```python
from build123d import *

# Parameters (mm, degrees)
CROQUIS1_W              = 100
CROQUIS1_H              = 150
SALIENTE_EXTRUIR1_DEPTH = 2
CROQUIS5_W              = 100
CROQUIS5_H              = 150
CROQUIS5_W_2            = 94
CROQUIS5_H_2            = 144
SALIENTE_EXTRUIR3_DEPTH = 15
CROQUIS6_W              = 20
CROQUIS6_H              = 20
SALIENTE_EXTRUIR4_DEPTH = 17
CROQUIS4_R              = 2
CORTAR_EXTRUIR2_DEPTH   = 92.378334412
SALIENTE_EXTRUIR5_DEPTH = 7.5
CROQUIS8_W              = 127.938872722
CROQUIS8_H              = 211.588515632
CROQUIS8_W_2            = 100
CROQUIS8_H_2            = 150
CORTAR_EXTRUIR3_DEPTH   = 115.867495711
CORTAR_EXTRUIR4_DEPTH   = 7.5
CROQUIS10_W             = 60
CROQUIS10_H             = 1.5
CROQUIS10_W_2           = 1.5
CROQUIS10_H_2           = 110
SALIENTE_EXTRUIR6_DEPTH = 3
CROQUIS12_R             = 0.6
CORTAR_EXTRUIR5_DEPTH   = 2
CORTAR_EXTRUIR7_DEPTH   = 157.655827733


with BuildPart() as part:
    # Croquis1 → Saliente-Extruir1 (new body)
    with BuildSketch(Plane(origin=(0, 0, 0), x_dir=(1, 0, 0), z_dir=(0, 1, 0))):
        Rectangle(CROQUIS1_W, CROQUIS1_H)
    extrude(amount=SALIENTE_EXTRUIR1_DEPTH)

    # Croquis5 → Saliente-Extruir3 (add)
    with BuildSketch(Plane(origin=(0, 2, 0), x_dir=(1, 0, 0), z_dir=(0, 1, 0))):
        Rectangle(CROQUIS5_W, CROQUIS5_H)
        Rectangle(CROQUIS5_W_2, CROQUIS5_H_2, mode=Mode.SUBTRACT)
    extrude(amount=SALIENTE_EXTRUIR3_DEPTH)

    # Croquis6 → Saliente-Extruir4 (add)
    with BuildSketch(Plane.XZ):
        with Locations((-40, 65)):
            Rectangle(CROQUIS6_W, CROQUIS6_H)
        with Locations((-40, -65)):
            Rectangle(CROQUIS6_W, CROQUIS6_H)
        with Locations((40, -65)):
            Rectangle(CROQUIS6_W, CROQUIS6_H)
        with Locations((40, 65)):
            Rectangle(CROQUIS6_W, CROQUIS6_H)
    extrude(amount=-SALIENTE_EXTRUIR4_DEPTH)

    # Croquis4 → Cortar-Extruir2 (cut, through all)
    # profile 1 of 4: a face of its own
    with BuildSketch(Plane(origin=(0, 2, 0), x_dir=(1, 0, 0), z_dir=(0, 1, 0))):
        with BuildLine():
            Line((-44.924038765, 64.131759112), (-46.660520542, 73.979836642))
            ThreePointArc((-46.660520542, 73.979836642), (-42.604722665, 79.772116295), (-36.812443012, 75.716318418))
            Line((-36.812443012, 75.716318418), (-35.075961235, 65.868240888))
            ThreePointArc((-35.075961235, 65.868240888), (-39.131759112, 60.075961235), (-44.924038765, 64.131759112))
        make_face()
        with Locations(Location((-40, 65, 0), (0, 0, 90))):
            Circle(CROQUIS4_R, mode=Mode.SUBTRACT)
    # profile 2 of 4: a face of its own
    with BuildSketch(Plane(origin=(0, 2, 0), x_dir=(1, 0, 0), z_dir=(0, 1, 0))):
        with BuildLine():
            Line((44.924038765, -64.131759112), (46.660520542, -73.979836642))
            ThreePointArc((46.660520542, -73.979836642), (42.604722665, -79.772116295), (36.812443012, -75.716318418))
            Line((36.812443012, -75.716318418), (35.075961235, -65.868240888))
            ThreePointArc((35.075961235, -65.868240888), (39.131759112, -60.075961235), (44.924038765, -64.131759112))
        make_face()
        with Locations(Location((40, -65, 0), (0, 0, 90))):
            Circle(CROQUIS4_R, mode=Mode.SUBTRACT)
    # profile 3 of 4: a face of its own
    with BuildSketch(Plane(origin=(0, 2, 0), x_dir=(1, 0, 0), z_dir=(0, 1, 0))):
        with BuildLine():
            Line((44.924038765, 64.131759112), (46.660520542, 73.979836642))
            ThreePointArc((46.660520542, 73.979836642), (42.604722665, 79.772116295), (36.812443012, 75.716318418))
            Line((36.812443012, 75.716318418), (35.075961235, 65.868240888))
            ThreePointArc((35.075961235, 65.868240888), (39.131759112, 60.075961235), (44.924038765, 64.131759112))
        make_face()
        with Locations(Location((40, 65, 0), (0, 0, 90))):
            Circle(CROQUIS4_R, mode=Mode.SUBTRACT)
    # profile 4 of 4: a face of its own
    with BuildSketch(Plane(origin=(0, 2, 0), x_dir=(1, 0, 0), z_dir=(0, 1, 0))):
        with BuildLine():
            Line((-44.924038765, -64.131759112), (-46.660520542, -73.979836642))
            ThreePointArc((-46.660520542, -73.979836642), (-42.604722665, -79.772116295), (-36.812443012, -75.716318418))
            Line((-36.812443012, -75.716318418), (-35.075961235, -65.868240888))
            ThreePointArc((-35.075961235, -65.868240888), (-39.131759112, -60.075961235), (-44.924038765, -64.131759112))
        make_face()
        with Locations(Location((-40, -65, 0), (0, 0, 90))):
            Circle(CROQUIS4_R, mode=Mode.SUBTRACT)
    extrude(amount=CORTAR_EXTRUIR2_DEPTH, mode=Mode.SUBTRACT)

    # Croquis7 → Saliente-Extruir5 (add)
    with BuildSketch(Plane(origin=(0, 2, 0), x_dir=(1, 0, 0), z_dir=(0, 1, 0))):
        with BuildLine():
            Line((35.075961235, 65.868240888), (39.187090394, 89.183612944))
            ThreePointArc((39.187090394, 89.183612944), (44.979370047, 93.239410821), (49.035167924, 87.447131167))
            Line((49.035167924, 87.447131167), (44.924038765, 64.131759112))
            ThreePointArc((44.924038765, 64.131759112), (39.131759112, 60.075961235), (35.075961235, 65.868240888))
        make_face()
        with BuildLine():
            Line((-44.924038765, 64.131759112), (-50.51627176, 95.846888427))
            ThreePointArc((-50.51627176, 95.846888427), (-46.460473883, 101.63916808), (-40.66819423, 97.583370203))
            Line((-40.66819423, 97.583370203), (-35.075961235, 65.868240888))
            ThreePointArc((-35.075961235, 65.868240888), (-39.131759112, 60.075961235), (-44.924038765, 64.131759112))
        make_face()
        with BuildLine():
            Line((-35.075961235, -65.868240888), (-36.812443012, -75.716318418))
            ThreePointArc((-36.812443012, -75.716318418), (-42.604722665, -79.772116295), (-46.660520542, -73.979836642))
            Line((-46.660520542, -73.979836642), (-44.924038765, -64.131759112))
            ThreePointArc((-44.924038765, -64.131759112), (-39.131759112, -60.075961235), (-35.075961235, -65.868240888))
        make_face()
        with BuildLine():
            Line((44.924038765, -64.131759112), (47.53565731, -78.942983887))
            ThreePointArc((47.53565731, -78.942983887), (43.479859434, -84.73526354), (37.68757978, -80.679465664))
            Line((37.68757978, -80.679465664), (35.075961235, -65.868240888))
            ThreePointArc((35.075961235, -65.868240888), (39.131759112, -60.075961235), (44.924038765, -64.131759112))
        make_face()
    extrude(amount=SALIENTE_EXTRUIR5_DEPTH)

    # Croquis8 → Cortar-Extruir3 (cut, through all)
    with BuildSketch(Plane.XZ):
        Rectangle(CROQUIS8_W, CROQUIS8_H)
        Rectangle(CROQUIS8_W_2, CROQUIS8_H_2, mode=Mode.SUBTRACT)
    extrude(amount=-CORTAR_EXTRUIR3_DEPTH, mode=Mode.SUBTRACT)

    # Croquis9 → Cortar-Extruir4 (cut)
    with BuildSketch(Plane(origin=(0, 17, 0), x_dir=(1, 0, 0), z_dir=(0, 1, 0))):
        with BuildLine():
            Line((-50, -74.5), (-50, -75))
            Line((-50, -75), (-44.511576947, -75))
            Line((-44.511576947, -75), (-44.511576947, -62.844617563))
            add(Edge.make_bspline(
                [(-50, -74.5), (-46.388295921, -69.021503378), (-44.511576947, -62.844617563)],
                knots=[0, 0, 0, 1, 1, 1], degree=2))
        make_face()
        with BuildLine():
            Line((50, -75), (44.511576947, -75))
            Line((44.511576947, -75), (44.511576947, -62.844617563))
            add(Edge.make_bspline(
                [(50, -74.5), (46.388295921, -69.021503378), (44.511576947, -62.844617563)],
                knots=[0, 0, 0, 1, 1, 1], degree=2))
            Line((50, -74.5), (50, -75))
        make_face()
        with BuildLine():
            Line((-50, 75), (-44.511576947, 75))
            Line((-44.511576947, 75), (-44.511576947, 62.844617563))
            add(Edge.make_bspline(
                [(-50, 74.5), (-46.388295921, 69.021503378), (-44.511576947, 62.844617563)],
                knots=[0, 0, 0, 1, 1, 1], degree=2))
            Line((-50, 74.5), (-50, 75))
        make_face()
        with BuildLine():
            Line((50, 75), (44.511576947, 75))
            Line((44.511576947, 75), (44.511576947, 62.844617563))
            add(Edge.make_bspline(
                [(50, 74.5), (46.388295921, 69.021503378), (44.511576947, 62.844617563)],
                knots=[0, 0, 0, 1, 1, 1], degree=2))
            Line((50, 74.5), (50, 75))
        make_face()
    extrude(amount=-CORTAR_EXTRUIR4_DEPTH, mode=Mode.SUBTRACT)

    # Croquis10 → Saliente-Extruir6 (add)
    with BuildSketch(Plane(origin=(0, 17, 0), x_dir=(1, 0, 0), z_dir=(0, 1, 0))):
        with Locations((0, 72.75)):
            Rectangle(CROQUIS10_W, CROQUIS10_H)
        with Locations((0, -72.75)):
            Rectangle(CROQUIS10_W, CROQUIS10_H)
        with Locations((-47.75, 0)):
            Rectangle(CROQUIS10_W_2, CROQUIS10_H_2)
        with Locations((47.75, 0)):
            Rectangle(CROQUIS10_W_2, CROQUIS10_H_2)
    extrude(amount=SALIENTE_EXTRUIR6_DEPTH)

    # Croquis12 → Cortar-Extruir5 (cut)
    with BuildSketch(Plane(origin=(0, 17, 0), x_dir=(1, 0, 0), z_dir=(0, 1, 0))):
        with Locations(Location((-40, -65, 0), (0, 0, 270))):
            Circle(CROQUIS12_R)
        with Locations(Location((-40, 65, 0), (0, 0, 90))):
            Circle(CROQUIS12_R)
        with Locations(Location((40, 65, 0), (0, 0, 270))):
            Circle(CROQUIS12_R)
        with Locations(Location((40, -65, 0), (0, 0, 90))):
            Circle(CROQUIS12_R)
    extrude(amount=-CORTAR_EXTRUIR5_DEPTH, mode=Mode.SUBTRACT)

    # Croquis17 → Revolución4 (revolve)
    with BuildSketch(Plane(origin=(-12.5, 0, -12.5), x_dir=(-0.7071067811865475, 0, 0.7071067811865476), z_dir=(-0.7071067811865476, 0, -0.7071067811865475)), mode=Mode.PRIVATE) as revoluci_n4_sk:
        Polygon((-74.388347648, 5.812970012), (-139.644463954, -21.860187069), (-143.51805142, -12.725874225), (-138.914857092, -10.773797899), (-136.962780767, -15.376992227), (-77.121254504, 10), align=None)
    revoluci_n4 = revolve(revoluci_n4_sk.sketch.rotate(Axis((40.100505063, 5.812970012, -65.100505063), (0.6509899848797962, -0.3904152650350718, -0.6509899848797963)), 90), axis=Axis((40.100505063, 5.812970012, -65.100505063), (0.6509899848797962, -0.3904152650350718, -0.6509899848797963)))

    # Simetría4: Revolución4 across plane
    add(revoluci_n4.mirror(Plane.XY))

    # Simetría5: Revolución4 across plane
    add(revoluci_n4.mirror(Plane(origin=(0, 0, 0), x_dir=(0, 0, 1), z_dir=(1, 0, 0))))

    # Simetría5 copy 1 sketch → Simetría5 copy 1 (revolve)
    with BuildSketch(Plane(origin=(12.5, 0, 12.5), x_dir=(0.7071067811865475, 0, -0.7071067811865476), z_dir=(0.7071067811865476, 0, 0.7071067811865475))):
        Polygon((-74.388347648, 5.812970012), (-139.644463954, -21.860187069), (-143.51805142, -12.725874225), (-138.914857092, -10.773797899), (-136.962780767, -15.376992227), (-77.121254504, 10), align=None)
    revolve(axis=Axis((-40.100505063, 5.812970012, 65.100505063), (-0.6509899848797962, -0.3904152650350718, 0.6509899848797963)))

    # Croquis19 → Cortar-Extruir7 (cut, through all)
    with BuildSketch(Plane(origin=(0, 9.5, 0), x_dir=(1, 0, 0), z_dir=(0, 1, 0))):
        Polygon((-43.417017803, -64.899000462), (-39.692445235, -68.264184449), (-41.99457515, -70.812172899), (-45.719147718, -67.446988912), align=None)
        Polygon((39.692445235, -68.264184449), (41.99457515, -70.812172899), (45.719147718, -67.446988912), (43.417017803, -64.899000462), align=None)
        Polygon((43.417017803, 64.899000462), (39.692445235, 68.264184449), (41.99457515, 70.812172899), (45.719147718, 67.446988912), align=None)
        Polygon((-39.692445235, 68.264184449), (-41.99457515, 70.812172899), (-45.719147718, 67.446988912), (-43.417017803, 64.899000462), align=None)
    extrude(amount=CORTAR_EXTRUIR7_DEPTH, mode=Mode.SUBTRACT)


solid = part.part
```
Work out the finished part from the listing and answer in its coordinate system (mm). A direction names the side the tool comes from. Coordinates: 2 decimals unless noted, no trailing zeros. Loops run counter-clockwise (first coordinate to the right, second up) from the corner with the lowest first, then second, coordinate; pieces in that order, holes last.
1) Section A-A (x = 23.5) is taken. Give the vertices of the cut face in (y, z).
Results:
outline: (0, -75) - (17, -75) - (17, -73.5) - (20, -73.5) - (20, -72) - (2, -72) - (2, 72) - (20, 72) - (20, 73.5) - (17, 73.5) - (17, 75) - (0, 75) - close
2) Flat-ended cylindrical pins translate along their axes: pin 1 (1.6 mm diameter, centred on x = 40, z = -65, fed in from -Y); pin 2 (4.5 mm diameter, centred on x = -42.5, y = 6.5, fed in from +Z); pin 3 (12 mm diameter, centred on y = 9, z = -63, fed in from -X). Find the tip coordinate at first contact, or state that the pin passes through.
Results:
pin 1: stops at y = 0
pin 2: stops at z = 75
pin 3: stops at x = -50
3) For a pull along Y with two mould halves and no side action, classify faces 1 (the flat face through (-85.558, -22.066, 104.125)), 2 (the flat face through (-30, 9, 63)), 3 (the flat face through (86.3, -21.99, 111.11)) as +Y half, -Y half, draft (parallel to the pull), parting line (faces both ways), or undercut.
Results:
face 1: undercut
face 2: draft
face 3: -Y half
4) For faces 4 (the cylindrical face through (39, 13.2, -60.1)), 5 (the flat face through (-86.3, -21.99, -111.11)), 6 (the flat face through (-80.076, -24.096, -108.39)), determine the directions among +Z, -Z, +X, -X, +Y, -Y from which every point of the face is accessible in a straight line to the end or side of a thin tool.
Results:
face 4: +Y
face 5: -Z, -X, -Y
face 6: none
5) Section B-B (z = 4.5) is taken. Give the vertices of the cut face in (x, y), plus the area to 3 significant figures.
Results:
outline: (-50, 0) - (50, 0) - (50, 17) - (48.5, 17) - (48.5, 20) - (47, 20) - (47, 2) - (-47, 2) - (-47, 20) - (-48.5, 20) - (-48.5, 17) - (-50, 17) - close
area: 299 mm2
6) Consider probe 1 along Z at (x, y) = (6, 11.5); probe 2 along X at (y, z) = (8, -45); probe 3 along Y at (x, z) = (43.5, -11.5). Determine where each line is inside the solid, lowest interval first.
Results:
probe 1: z = -75 to -72, 72 to 75
probe 2: x = -50 to -47, 47 to 50
probe 3: y = 0 to 2
7) Section C-C (y = -8) is taken. Give the number of separate pieces and of enclosed holes in the cut face, plus the area to 3 significant figures.
Results:
separate pieces: 4
enclosed holes: 0
area: 780 mm2
